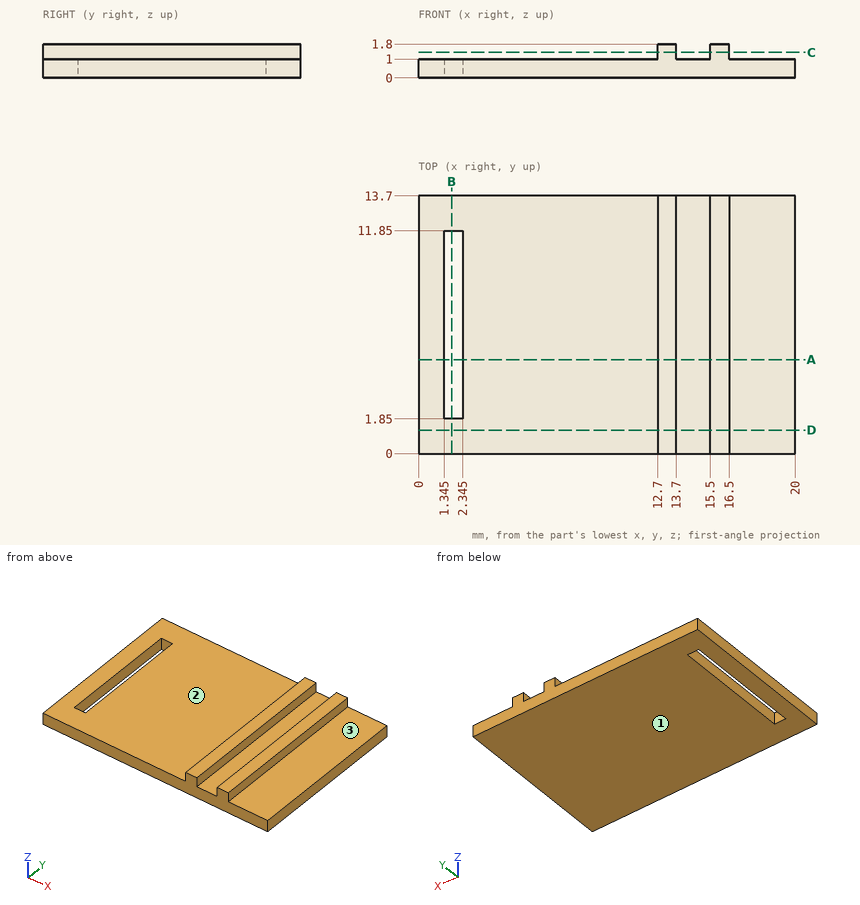
The drawing under review shows one solid part. Ordinate dimensions are in mm from its lowest x, y, z. A direction names the side the tool comes from. Round coordinates to 2 decimals unless told otherwise and drop trailing zeros. Write each loop counter-clockwise with the first axis right and the second up, starting at its lowest first coordinate (ties: lowest second). Pieces come first, ordered by that corner, then holes.
(1) We need section D-D on y = 1.25. Give the boundary of the cut face in (x, z).
(2) We need section C-C on z = 1.35. Give the boundary of the cut face in (x, y), and give its area (3 significant figures).
(3) Insertion check: pin 1 (0.9 mm diameter, centred on y = 5, z = 1.5, fed in from +X); pin 2 (2 mm diameter, centred on x = 5.5, y = 12.5, fed in from +Z). Each pin has a flat end and moves straight along its axis. Give the tip position at first contact, or say it passes through.
(4) We need section B-B on x = 1.75. Give the boundary of the cut face in (y, z), and give its area (3 significant figures).
(5) We need section A-A on y = 5. Give the boundary of the cut face in (x, z) (3 decimals), and give its area (3 significant figures).
(6) Machinability: for the marked faces 1, 2 and 3, which of the approach directions +Z, -Z, +X, -X, +Y, -Y give a long, thin tool a straight path to every point of the face, cutting with its end or side? Answer none if there is none.
(7) Wall thickness on L1, parallel to X at y = 6, z = 1.4; L2, parallel to X at y = 9, z = 0.4 (3 decimals); L3, parallel to Y at x = 1.5, z = 0.9: over which ranges is each line inside the solid? List them lowest first.
Findings below:
1. outline: (0, 0) - (20, 0) - (20, 1) - (16.5, 1) - (16.5, 1.8) - (15.5, 1.8) - (15.5, 1) - (13.7, 1) - (13.7, 1.8) - (12.7, 1.8) - (12.7, 1) - (0, 1) - close
2. outline: (12.7, 0) - (13.7, 0) - (13.7, 13.7) - (12.7, 13.7) - close; (15.5, 0) - (16.5, 0) - (16.5, 13.7) - (15.5, 13.7) - close
2. area: 27.4 mm2
3. pin 1: stops at x = 16.5
3. pin 2: stops at z = 1
4. outline: (0, 0) - (1.85, 0) - (1.85, 1) - (0, 1) - close; (11.85, 0) - (13.7, 0) - (13.7, 1) - (11.85, 1) - close
4. area: 3.70 mm2
5. outline: (0, 0) - (1.345, 0) - (1.345, 1) - (0, 1) - close; (2.345, 0) - (20, 0) - (20, 1) - (16.5, 1) - (16.5, 1.8) - (15.5, 1.8) - (15.5, 1) - (13.7, 1) - (13.7, 1.8) - (12.7, 1.8) - (12.7, 1) - (2.345, 1) - close
5. area: 20.6 mm2
6. face 1: -Z, +X, -X, +Y, -Y
6. face 2: +Z, -X, +Y, -Y
6. face 3: +Z, +X, +Y, -Y
7. L1: x = 12.7 to 13.7, 15.5 to 16.5
7. L2: x = 0 to 1.345, 2.345 to 20
7. L3: y = 0 to 1.85, 11.85 to 13.7
